```python
from build123d import *

# Parameters (mm, degrees)
BOSS_EXTRUDE1_DEPTH = 14.5
SKETCH2_R           = 0.75
CUT_EXTRUDE1_DEPTH  = 18.381785246


with BuildPart() as part:
    # Sketch1 → Boss-Extrude1 (new body)
    with BuildSketch(Plane(origin=(0, 0, 0), x_dir=(1, 0, 0), z_dir=(0, 1, 0))):
        Polygon((-3.622872939, 6.275), (-7.245745878, 0), (-3.622872939, -6.275), (3.622872939, -6.275), (7.245745878, 0), (3.622872939, 6.275), align=None)
        Polygon((4.156921938, 0), (2.078460969, 3.6), (-2.078460969, 3.6), (-4.156921938, 0), (-2.078460969, -3.6), (2.078460969, -3.6), align=None, mode=Mode.SUBTRACT)
    extrude(amount=BOSS_EXTRUDE1_DEPTH)

    # Sketch2 → Cut-Extrude1 (cut, through all)
    with BuildSketch(Plane(origin=(0, 14.5, 0), x_dir=(1, 0, 0), z_dir=(0, 1, 0))):
        with Locations((-2.078460969, 3.6)):
            Circle(SKETCH2_R)
        with Locations((2.078460969, 3.6)):
            Circle(SKETCH2_R)
        with Locations((4.156921938, 0)):
            Circle(SKETCH2_R)
        with Locations((2.078460969, -3.6)):
            Circle(SKETCH2_R)
        with Locations((-2.078460969, -3.6)):
            Circle(SKETCH2_R)
        with Locations((-4.156921938, 0)):
            Circle(SKETCH2_R)
    extrude(amount=-CUT_EXTRUDE1_DEPTH, mode=Mode.SUBTRACT)


solid = part.part
```
The listing builds one solid part. Answer for the finished solid, in the listing's coordinates (mm). A direction names the side the tool comes from. Give positions to 0.01 mm unless a question says otherwise; leave off trailing zeros. Write each loop counter-clockwise with the first axis right and the second up, starting at its lowest first coordinate (ties: lowest second). Pieces come first, ordered by that corner, then holes. Notation, with made-up numbers: (32, 51) -> (70, 51) arc R5 cw to (70, 55) -> close; hole circle Ø10 at (-15.75, -6.5). An arc over 180 degrees is marked (long way). Use one line per item in the form item = value.
1) For a pull along Z with two mould halves and no side action, classify faces 3 (the flat face through (5.46, 7.15, -3.09)), 4 (the flat face through (0, 7, -3.6)), 5 (the flat face through (-5.46, 7.15, 3.09)), 6 (the cylindrical face through (4.907, 7.352, 0.022)) as +Z half, -Z half, draft (parallel to the pull), parting line (faces both ways), or undercut.
Result:
face_3 = -Z half
face_4 = undercut
face_5 = +Z half
face_6 = undercut
2) A tool of negligible diameter and unlimited length cuts with its end or side. For faces 1 (the flat face through (0, 7, 3.6)), 2 (the flat face through (-5.4, 7.1, -3.2)), from which of +Z, -Z, +X, -X, +Y, -Y can it reach the whole face along a straight path? Write none if from no direction.
Result:
face_1 = +Y, -Y
face_2 = -Z, -X, +Y, -Y
3) Section B-B on y = 7.5 is taken. Write down the section's boundary in (x, z) (3 decimals).
Result:
outline = (-7.246, 0) -> (-3.623, -6.275) -> (3.623, -6.275) -> (7.246, 0) -> (3.623, 6.275) -> (-3.623, 6.275) -> close; hole (-3.782, -0.65) -> (-2.453, -2.95) arc R0.75 ccw (long way) to (-1.328, -3.6) -> (1.328, -3.6) arc R0.75 ccw (long way) to (2.453, -2.95) -> (3.782, -0.65) arc R0.75 ccw (long way) to (3.782, 0.65) -> (2.453, 2.95) arc R0.75 ccw (long way) to (1.328, 3.6) -> (-1.328, 3.6) arc R0.75 ccw (long way) to (-2.453, 2.95) -> (-3.782, 0.65) arc R0.75 ccw (long way) to start
4) Section C-C on z = -2 is taken. Write down the section's boundary in (x, y).
Result:
outline = (-6.09, 0) -> (-3, 0) -> (-3, 14.5) -> (-6.09, 14.5) -> close; (3, 0) -> (6.09, 0) -> (6.09, 14.5) -> (3, 14.5) -> close
5) Each of these flat-tipped pins is pushed along its axis until it touches: P1, Ø3, axis at y = 7, z = -3.5, coming from the -X side; P2, Ø1.5, axis at x = 5, y = 2.5, coming from the -Z side. Where does it stop, or does it pass through?
Result:
P1 = -6.09
P2 = -5.19
6) Straight lines are drawn through the part: probe 1 along X at (y, z) = (1.75, -4); probe 2 along Z at (x, y) = (0, 2.5) (3 decimals); probe 3 along Z at (x, y) = (-3, 3) (3 decimals). For each, find the intervals that lie inside material, in ascending order.
Result:
probe_1 = -4.94 to -2.71, -1.44 to 1.44, 2.71 to 4.94
probe_2 = -6.275 to -3.6, 3.6 to 6.275
probe_3 = -6.275 to -2.004, 2.004 to 6.275
7) Section A-A on x = 0.5 is taken. Write down the section's boundary in (y, z) (3 decimals), plus the area to 3 significant figures.
Result:
outline = (0, -6.275) -> (14.5, -6.275) -> (14.5, -3.6) -> (0, -3.6) -> close; (0, 3.6) -> (14.5, 3.6) -> (14.5, 6.275) -> (0, 6.275) -> close
area = 77.6 mm²
